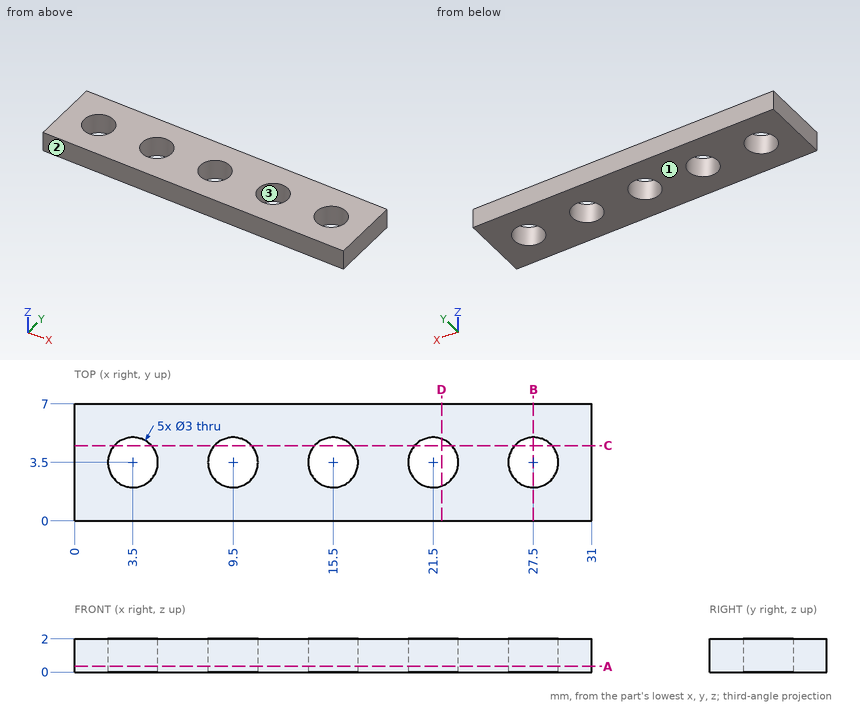
Check sheet for the drawn part. Datum: minimum x, y, z corner. Units: mm. Give positions to 0.01 mm unless a question says otherwise; leave off trailing zeros. Loops run counter-clockwise (first coordinate to the right, second up) from the corner with the lowest first, then second, coordinate; pieces in that order, holes last.
1) Depth check by flat-ended pin: pin 1 Ø2.5 at (x, y) = (9.5, 3.5) entering from +Z. Enter the tip coordinate at first touch or a pass-through.
2) Sectioned sample at B-B, the plane x = 27.5. Enter the section's corners in (y, z).
3) Sectioned sample at A-A, the plane z = 0.35. Enter the section's corners in (x, y), then the cut area to 3 significant figures.
4) Sectioned sample at C-C, the plane y = 4.5. Enter the section's corners in (x, z).
5) Thickness scan on line 1 along Y through (x, z) = (21.5, 0.6); line 2 along X through (y, z) = (3.25, 1.3); line 3 along Y through (x, z) = (22.5, 0.3). Record the ranges inside material, lowest first.
6) Sectioned sample at D-D, the plane x = 22. Enter the section's corners in (y, z), then the cut area to 3 significant figures.
7) Draft check along Y on the marked faces 1, 2 and 3. Enter one of: pulls with the +Y half, pulls with the -Y half, needs draft (parallel to the pull), parting line crosses it, or undercut.
Answers:
1. pin 1: passes through
2. outline: (0, 0) - (2, 0) - (2, 2) - (0, 2) - close; (5, 0) - (7, 0) - (7, 2) - (5, 2) - close
3. outline: (0, 0) - (31, 0) - (31, 7) - (0, 7) - close; hole circle Ø3 at (3.5, 3.5); hole circle Ø3 at (9.5, 3.5); hole circle Ø3 at (15.5, 3.5); hole circle Ø3 at (21.5, 3.5); hole circle Ø3 at (27.5, 3.5)
3. area: 182 mm2
4. outline: (0, 0) - (2.38, 0) - (2.38, 2) - (0, 2) - close; (4.62, 0) - (8.38, 0) - (8.38, 2) - (4.62, 2) - close; (10.62, 0) - (14.38, 0) - (14.38, 2) - (10.62, 2) - close; (16.62, 0) - (20.38, 0) - (20.38, 2) - (16.62, 2) - close; (22.62, 0) - (26.38, 0) - (26.38, 2) - (22.62, 2) - close; (28.62, 0) - (31, 0) - (31, 2) - (28.62, 2) - close
5. line 1: y = 0 to 2, 5 to 7
5. line 2: x = 0 to 2.02, 4.98 to 8.02, 10.98 to 14.02, 16.98 to 20.02, 22.98 to 26.02, 28.98 to 31
5. line 3: y = 0 to 2.38, 4.62 to 7
6. outline: (0, 0) - (2.09, 0) - (2.09, 2) - (0, 2) - close; (4.91, 0) - (7, 0) - (7, 2) - (4.91, 2) - close
6. area: 8.34 mm2
7. face 1: needs draft
7. face 2: pulls with the -Y half
7. face 3: undercut
